Design review of the part built by this model. Coordinates are the model's own, in mm. A direction names the side the tool comes from. Give positions to 0.01 mm unless a question says otherwise; leave off trailing zeros. Loops run counter-clockwise (first coordinate to the right, second up) from the corner with the lowest first, then second, coordinate; pieces in that order, holes last. Notation, with made-up numbers: M 45,1 L 79,1 A36 cw 79,40 Z; hole C 47,22.5 d11. An arc over 180 degrees is marked long. Use one line per item in the form item = value. Start each with the question number.
from build123d import *

# Parameters (mm, degrees)
SKETCH1_W           = 125
SKETCH1_H           = 130
BOSS_EXTRUDE1_DEPTH = 2
SKETCH2_W           = 129
SKETCH2_H           = 134
SKETCH2_W_2         = 125
SKETCH2_H_2         = 130
BOSS_EXTRUDE2_DEPTH = 30
SKETCH3_R           = 2.75
BOSS_EXTRUDE3_DEPTH = 4
SKETCH4_R           = 1.75
CUT_EXTRUDE1_DEPTH  = 4
SKETCH5_W           = 11
SKETCH5_H           = 2
CUT_EXTRUDE2_DEPTH  = 5
SKETCH6_R           = 3
SKETCH6_R_2         = 5
CUT_EXTRUDE3_DEPTH  = 5


with BuildPart() as part:
    # Sketch1 → Boss-Extrude1 (new body)
    with BuildSketch(Plane(origin=(0, 0, 0), x_dir=(1, 0, 0), z_dir=(0, 1, 0))):
        with Locations((62.5, 65)):
            Rectangle(SKETCH1_W, SKETCH1_H)
    extrude(amount=BOSS_EXTRUDE1_DEPTH)

    # Sketch2 → Boss-Extrude2 (add)
    with BuildSketch(Plane.XZ):
        with Locations((62.5, -65)):
            Rectangle(SKETCH2_W, SKETCH2_H)
        with Locations((62.5, -65)):
            Rectangle(SKETCH2_W_2, SKETCH2_H_2, mode=Mode.SUBTRACT)
    extrude(amount=-BOSS_EXTRUDE2_DEPTH)

    # Sketch3 → Boss-Extrude3 (add)
    with BuildSketch(Plane(origin=(0, 2, 0), x_dir=(1, 0, 0), z_dir=(0, 1, 0))):
        with Locations((35, 68)):
            Circle(SKETCH3_R)
        with Locations((81, 68)):
            Circle(SKETCH3_R)
        with Locations((81, 2)):
            Circle(SKETCH3_R)
        with Locations((35, 2)):
            Circle(SKETCH3_R)
    extrude(amount=BOSS_EXTRUDE3_DEPTH)

    # Sketch4 → Cut-Extrude1 (cut)
    with BuildSketch(Plane(origin=(0, 6, 0), x_dir=(1, 0, 0), z_dir=(0, 1, 0))):
        with Locations((81, 2)):
            Circle(SKETCH4_R)
        with Locations((35, 2)):
            Circle(SKETCH4_R)
        with Locations((35, 68)):
            Circle(SKETCH4_R)
        with Locations((81, 68)):
            Circle(SKETCH4_R)
    extrude(amount=-CUT_EXTRUDE1_DEPTH, mode=Mode.SUBTRACT)

    # Sketch5 → Cut-Extrude2 (cut)
    with BuildSketch(Plane(origin=(0, 20.5, 0), x_dir=(1, 0, 0), z_dir=(0, 1, 0))):
        with Locations((58, -1)):
            Rectangle(SKETCH5_W, SKETCH5_H)
    extrude(amount=CUT_EXTRUDE2_DEPTH, mode=Mode.SUBTRACT)

    # Sketch6 → Cut-Extrude3 (cut)
    with BuildSketch(Plane(origin=(0, 0, 0), x_dir=(-1, 0, 0), z_dir=(0, 0, -1))):
        with Locations((-17.024516763, 17.032581473)):
            Circle(SKETCH6_R)
        with Locations((-111.272952747, 14.032581473)):
            Circle(SKETCH6_R_2)
    extrude(amount=-CUT_EXTRUDE3_DEPTH, mode=Mode.SUBTRACT)


solid = part.part
Q1. Take a section at A-A on x = 111.5. Give the boundary of the cut face in (y, z).
Q2. Clearance check with flat-ended pins moving along their axes: pin 1 Ø4 at (x, z) = (35, -68) entering from +Y; pin 2 Ø5 at (x, z) = (46.5, -59.5) entering from +Y. State where each tip first meets the part, or that it passes through.
Q3. Wall thickness on probe 1 along Z at (x, y) = (35, 3.5); probe 2 along X at (y, z) = (4.65, -2); probe 3 along X at (y, z) = (18, -5): over which ranges is each line inside the solid? List them lowest first.
Q4. Take a section at C-C on y = 4. Give the boundary of the cut face in (x, z), plus the area to 3 significant figures.
Q5. The part is to be moulded in two halves that separate along X. For faces 1 (the flat face through (-2, 15, -66)), 2 (the flat face through (62, 0, -64)), 3 (the flat face through (62, 16, 0)), say which applies: pulls with the +X half, pulls with the -X half, needs draft (parallel to the pull), parting line crosses it, or undercut.
Q6. Take a section at D-D on x = 75.5. Give the boundary of the cut face in (y, z), plus the area to 3 significant figures.
Q7. Take a section at B-B on z = -85. Give the boundary of the cut face in (x, y).
Q8. For faces 4 (the flat face through (81, 6, -66)), 5 (the flat face through (62, 15, -132)), 6 (the cylindrical face through (20.02, 17.16, 0.99)), list the 3-axis set-ups (+Z, -Z, +X, -X, +Y, -Y) from which the entire face can be reached by the end or side of a thin tool; tool diameter is ignored.
Response values:
q1.outline = M 0,-132 L 30,-132 L 30,-130 L 2,-130 L 2,0 L 9.04,0 L 9.04,2 L 0,2 Z; M 19.03,0 L 30,0 L 30,2 L 19.03,2 Z
q2.pin_1 = 6
q2.pin_2 = 2
q3.probe_1 = -132 to -130, -70.75 to -69.75, -66.25 to -65.25, -4.75 to -3.75, -0.25 to 2
q3.probe_2 = -2 to 0, 32.25 to 33.25, 36.75 to 37.75, 78.25 to 79.25, 82.75 to 83.75, 125 to 127
q3.probe_3 = -2 to 0, 125 to 127
q4.outline = M -2,-132 L 127,-132 L 127,2 L -2,2 Z; C 35,-68 d5.5; C 81,-68 d5.5; hole M 0,-130 L 125,-130 L 125,0 L 82.89,0 A2.75 cw long 79.11,0 L 36.89,0 A2.75 cw long 33.11,0 L 0,0 Z; hole C 35,-68 d3.5; hole C 35,-2 d3.5; hole C 81,-68 d3.5; hole C 81,-2 d3.5
q4.area = 1,090 mm^2
q5.face_1 = pulls with the -X half
q5.face_2 = needs draft
q5.face_3 = undercut
q6.outline = M 0,-132 L 30,-132 L 30,-130 L 2,-130 L 2,0 L 30,0 L 30,2 L 0,2 Z
q6.area = 380 mm^2
q7.outline = M -2,0 L 127,0 L 127,30 L 125,30 L 125,2 L 0,2 L 0,30 L -2,30 Z
q8.face_4 = +Y
q8.face_5 = -Z, +X, -X, +Y, -Y
q8.face_6 = +Z
